Source: CAD feature listing. Evaluate the final solid. Frame: model axes, mm. Face numbers are marked on the shaded views. A direction names the side the tool comes from. Give positions to 0.01 mm unless a question says otherwise; leave off trailing zeros. Loops run counter-clockwise (first coordinate to the right, second up) from the corner with the lowest first, then second, coordinate; pieces in that order, holes last. Notation, with made-up numbers: (83, -27) - (91, -27) arc R11 ccw to (91, -19) - close; hole circle Ø7 at (-5, -19). An arc over 180 degrees is marked (long way). Write each question's results on one line, items separated by ' | '. Start each with the question number.
(1) Cut plane B-B on y = 13.5. Return the cut outline in (x, z).
(2) Cut plane D-D on y = 29. Return the cut outline in (x, z).
(3) Material intervals for line 1 along Z through (x, y) = (-45.5, 3); line 2 along Z through (x, y) = (-38, 1.2); line 3 along X through (y, z) = (2.5, 14), sorted ascending. Write a range as [from, to].
(4) Cut plane A-A on x = 44. Return the cut outline in (y, z).
(5) Reachability of the marked faces 5, 6 and 7 from +Z, -Z, +X, -X, +Y, -Y: full face, straight path, thin tool, end or side. Return the list, or none.
(6) Cut plane C-C on z = 23.25. Return the cut outline in (x, y), then the cut area to 3 significant figures.
(7) Contact query for flat-ended pins moving along their axis: pin 1 (5.5 mm diameter, centred on x = -2, z = 18.5, fed in from -Y); pin 2 (5 mm diameter, centred on x = 1, z = 16.5, fed in from -Y); pin 3 (10 mm diameter, centred on x = 3.5, z = 22, fed in from -Y); pin 4 (3.5 mm diameter, centred on x = 0, z = 15, fed in from -Y). Output: stop coordinate, or through.
(8) Pull-direction query (X, two-part tool) for the marked faces 1, 2, 3 and 4; classes: pulls with the +X half, pulls with the -X half, needs draft (parallel to the pull), parting line crosses it, or undercut.
from build123d import *

# Parameters (mm, degrees)
F1_DEPTH = 30
F2_W     = 23
F2_H     = 12
F2_R     = 0.75
F3_DEPTH = 25
F4_R     = 10
F5_R     = 3
F6_DEPTH = 25
F7_DEPTH = 5


# Not quite as in the source:
# - a feature names something its author has since deleted; it is built from what else it names


with BuildPart() as f1:
    # F0 (on Top) → F1 (new body)
    with BuildSketch(Plane.XY):
        Polygon((30, 4), (10, 31), (-10, 31), (-30, 4), (-70, 4), (-70, 0), (-28, 0), (-10, 21), (10, 21), (28, 0), (70, 0), (70, 4), align=None)
    extrude(amount=F1_DEPTH)

    # F2 (on face) → F3 (cut)
    with BuildSketch(Plane(origin=(0, 4, 0), x_dir=(-1, 0, 0), z_dir=(0, 1, 0))):
        with Locations((52.5, 15)):
            Rectangle(F2_W, F2_H)
        with Locations((-52.5, 15)):
            Rectangle(F2_W, F2_H)
        with Locations((-38, 15)):
            Circle(F2_R)
        with Locations((-67, 15)):
            Circle(F2_R)
        with Locations((38, 15)):
            Circle(F2_R)
        with Locations((67, 15)):
            Circle(F2_R)
    extrude(amount=-F3_DEPTH, mode=Mode.SUBTRACT)

    # F4
    f4_edges = [f1.edges().sort_by_distance(p)[0] for p in [
        (-70, 2, 30),
        (-70, 2, 0),
        (70, 2, 30),
        (70, 2, 0),
        (30, 4, 15),
        (-30, 4, 15),
        (-10, 31, 15),
        (10, 31, 15),
        (-28, 0, 15),
        (-10, 21, 15),
        (10, 21, 15),
        (28, 0, 15),
    ]]
    fillet(f4_edges, radius=F4_R)

    # F5 (on face) → F6 (cut)
    with BuildSketch(Plane.XZ.offset(-21)):
        with Locations((0, 15)):
            Circle(F5_R)
    extrude(amount=-F6_DEPTH, mode=Mode.SUBTRACT)

    # F5 (on face) → F7 (cut)
    with BuildSketch(Plane.XZ.offset(-21)):
        Polygon((0, 9.1687622812), (5.05, 12.0843811406), (5.05, 17.9156188594), (0, 20.8312377188), (-5.05, 17.9156188594), (-5.05, 12.0843811406), align=None)
        with Locations((0, 15)):
            Circle(F5_R, mode=Mode.SUBTRACT)
    extrude(amount=-F7_DEPTH, mode=Mode.SUBTRACT)


solid = f1.part
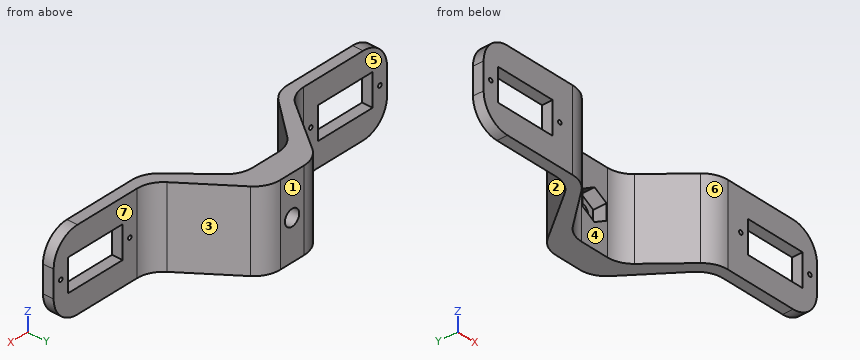
Ans:
1) outline: (-22.96, 0) - (-16.43, 0) - (-16.43, 30) - (-22.96, 30) - close; (16.43, 0) - (22.96, 0) - (22.96, 30) - (16.43, 30) - close
2) outline: (-10.96, 0) - (10.96, 0) - (10.96, 30) - (-10.96, 30) - close; hole circle Ø6 at (0, 15)
3) line 1: [0, 9], [21, 30] | line 2: [0, 14.25], [15.75, 30] | line 3: [-70, -64], [-41, -25.98], [25.98, 41], [64, 70]
4) outline: (0, 0) - (4, 0) - (4, 9) - (0, 9) - close; (0, 21) - (4, 21) - (4, 30) - (0, 30) - close
5) face 5: +Z, -Z, -X, +Y | face 6: +Z, -Z, -Y | face 7: +Z, -Z, +X, +Y
6) outline: (-69.46, 0) - (-32.6, 0) arc R10 ccw to (-25.01, 3.49) - (-12.99, 17.51) arc R10 cw to (-5.4, 21) - (5.4, 21) arc R10 cw to (12.99, 17.51) - (25.01, 3.49) arc R10 ccw to (32.6, 0) - (69.46, 0) - (69.46, 4) - (35.04, 4) arc R10 cw to (27, 8.05) - (13, 26.95) arc R10 ccw to (4.96, 31) - (-4.96, 31) arc R10 ccw to (-13, 26.95) - (-27, 8.05) arc R10 cw to (-35.04, 4) - (-69.46, 4) - close | area: 838 mm^2
7) pin 1: y = 21 | pin 2: y = 26 | pin 3: y = 20.51 | pin 4: through
8) face 1: needs draft | face 2: pulls with the -X half | face 3: pulls with the +X half | face 4: undercut
